```python
from build123d import *

# Parameters (mm, degrees)
SKETCH1_W               = 50
SKETCH1_H               = 60
BASE_FLANGE1_DEPTH      = 0.7366
SKETCHED_START          = -25
SKETCHED_BEND1_DEPTH    = 50
SKETCHED_BEND1_2_DEPTH  = 50
CUT_EXTRUDE1_DEPTH      = 54.090671485
CUT_EXTRUDE1_DEPTH_BACK = 54.090671485
SKETCH8_R               = 4


# Read off the part's stored shape, not the designer's step: Sketched Bend1
# Sheet-metal steps are written as plain solids
with BuildPart() as part:
    # Sketch1 → Base-Flange1 (new body)
    with BuildSketch(Plane.XY):
        Rectangle(SKETCH1_W, SKETCH1_H)
    extrude(amount=-BASE_FLANGE1_DEPTH)

    # Sketched Bend1 outline → Sketched Bend1 (cut)
    with BuildSketch(Plane.YZ.offset(SKETCHED_START)):
        with BuildLine():
            ThreePointArc((9.066731634, -0.7366), (8.062794494, -0.545798456), (7.198850599, 0))
            Line((7.198850599, 0), (-30, 0))
            Line((-30, 0), (-30, -0.7366))
            Line((-30, -0.7366), (9.066731634, -0.7366))
        make_face()
    extrude(amount=SKETCHED_BEND1_DEPTH, mode=Mode.SUBTRACT)

    # Sketched Bend1 2 outline → Sketched Bend1 2 (add)
    with BuildSketch(Plane.YZ.offset(SKETCHED_START)):
        with BuildLine():
            Line((13.163214519, 36.74984988), (12.437805129, 36.877759128))
            Line((12.437805129, 36.877759128), (6.371706737, 2.475205603))
            ThreePointArc((6.371706737, 2.475205603), (6.471218519, 1.132652762), (7.198850599, 0))
            Line((7.198850599, 0), (9.066731634, 0))
            ThreePointArc((9.066731634, 0), (7.534642748, 0.714424781), (7.097116128, 2.347296355))
            Line((7.097116128, 2.347296355), (13.163214519, 36.74984988))
        make_face()
    extrude(amount=SKETCHED_BEND1_2_DEPTH)

    # Sketch8 → Cut-Extrude1 (cut, two sides: drawn at the far end of the back side and taken through both)
    with BuildSketch(Plane(origin=(0, 0.074278928, 0.849012035), x_dir=(1, 0, 0), z_dir=(0, 0.17364817766693058, 0.984807753012208)).offset(-CUT_EXTRUDE1_DEPTH_BACK)):
        with Locations(Location((0, 22.91937018, 0), (0, 0, 90))):
            Circle(SKETCH8_R)
    extrude(amount=CUT_EXTRUDE1_DEPTH + CUT_EXTRUDE1_DEPTH_BACK, mode=Mode.SUBTRACT)


solid = part.part
```
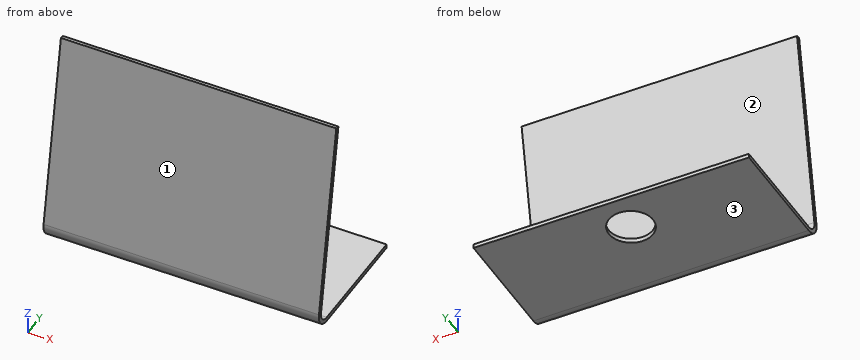
Can you work these out from the model? Positions are in its coordinate system, mm. Face numbers are marked on the shaded views. Coordinates: 2 decimals unless noted, no trailing zeros. Loops run counter-clockwise (first coordinate to the right, second up) from the corner with the lowest first, then second, coordinate; pieces in that order, holes last.
1) Imagine slicing it at C-C on y = 15. List the corners of the cut face in (x, z) for me, plus the area to 3 significant figures.
2) Imagine slicing it at A-A on x = 6. List the corners of the cut face in (y, z) for me, plus the area to 3 significant figures.
3) Imagine slicing it at B-B on y = 11.75. List the corners of the cut face in (x, z) for me.
4) Imagine slicing it at D-D on z = 12. List the corners of the cut face in (x, y) for me, plus the area to 3 significant figures.
5) For pin 1 (1.5 mm diameter, centred on x = 11.5, y = 21.5, fed in from +Z), with a flat end and sliding along its axis, tell me the tip position at first contact or that it passes through.
6) I need wall thicknesses on probe 1 along Z at (x, y) = (13, 27); probe 2 along Y at (x, z) = (-18, 24.5); probe 3 along Y at (x, z) = (-10, 28.5). Which ranges of each line are inside material? Lowest first, please.
7) Thinking about a two-plate mould opening in Z: for the marked faces 1, 2 and 3, which applies, pulls with the +Z half, pulls with the -Z half, needs draft (parallel to the pull), parting line crosses it, or undercut?
Completed:
1. outline: (-25, -0.74) - (25, -0.74) - (25, 0) - (-25, 0) - close
1. area: 36.8 mm2
2. outline: (6.37, 2.48) arc R2.74 ccw to (9.07, -0.74) - (30, -0.74) - (30, 0) - (9.07, 0) arc R2 cw to (7.1, 2.35) - (13.16, 36.75) - (12.44, 36.88) - close
2. area: 44.2 mm2
3. outline: (-25, -0.74) - (25, -0.74) - (25, 0) - (-25, 0) - close; (-25, 28.74) - (25, 28.74) - (25, 32.98) - (-25, 32.98) - close
4. outline: (-25, 8.05) - (25, 8.05) - (25, 8.8) - (-25, 8.8) - close
4. area: 37.4 mm2
5. pin 1: stops at z = 0
6. probe 1: z = -0.74 to 0
6. probe 2: y = 10.26 to 11
6. probe 3: y = 10.96 to 11.71
7. face 1: pulls with the +Z half
7. face 2: undercut
7. face 3: pulls with the -Z half
